from build123d import *

# Parameters (mm, degrees)
CROQUIS1_W              = 190
CROQUIS1_H              = 115.4
SALIENTE_EXTRUIR1_DEPTH = 3
CROQUIS2_R              = 1.6
CORTAR_EXTRUIR1_DEPTH   = 5
CROQUIS4_R              = 1.1
CORTAR_EXTRUIR3_DEPTH   = 5
CROQUIS5_W              = 35.625
CROQUIS5_H              = 40
CORTAR_EXTRUIR4_DEPTH   = 5
REDONDEO1_R             = 3
REDONDEO2_R             = 3
REDONDEO3_R             = 3
REDONDEO4_R             = 3
CROQUIS7_R              = 1.6
CORTAR_EXTRUIR6_DEPTH   = 10
CROQUIS6_R              = 2.1
CORTAR_EXTRUIR7_DEPTH   = 3


with BuildPart() as part:
    # Croquis1 → Saliente-Extruir1 (new body)
    with BuildSketch(Plane(origin=(0, 0, 0), x_dir=(1, 0, 0), z_dir=(0, 1, 0))):
        Rectangle(CROQUIS1_W, CROQUIS1_H)
    extrude(amount=SALIENTE_EXTRUIR1_DEPTH)

    # Croquis2 → Cortar-Extruir1 (cut)
    with BuildSketch(Plane(origin=(0, 3, 0), x_dir=(1, 0, 0), z_dir=(0, 1, 0))):
        with Locations(Location((-36.375, -51.1, 0), (0, 0, 270))):
            Circle(CROQUIS2_R)
        with Locations(Location((-36.375, -10.3, 0), (0, 0, 270))):
            Circle(CROQUIS2_R)
        with Locations(Location((34.375, -10.3, 0), (0, 0, 270))):
            Circle(CROQUIS2_R)
        with Locations(Location((34.375, -51.1, 0), (0, 0, 270))):
            Circle(CROQUIS2_R)
    extrude(amount=-CORTAR_EXTRUIR1_DEPTH, mode=Mode.SUBTRACT)

    # Croquis4 → Cortar-Extruir3 (cut)
    with BuildSketch(Plane(origin=(0, 3, 0), x_dir=(1, 0, 0), z_dir=(0, 1, 0))):
        with Locations(Location((-51.375, -50.7, 0), (0, 0, 270))):
            Circle(CROQUIS4_R)
        with Locations(Location((-51.375, -33.3, 0), (0, 0, 270))):
            Circle(CROQUIS4_R)
        with Locations(Location((51.375, -33.3, 0), (0, 0, 270))):
            Circle(CROQUIS4_R)
        with Locations(Location((51.375, -50.7, 0), (0, 0, 270))):
            Circle(CROQUIS4_R)
    extrude(amount=-CORTAR_EXTRUIR3_DEPTH, mode=Mode.SUBTRACT)

    # Croquis5 → Cortar-Extruir4 (cut)
    with BuildSketch(Plane(origin=(0, 3, 0), x_dir=(1, 0, 0), z_dir=(0, 1, 0))):
        with Locations((-77.1875, -37.7)):
            Rectangle(CROQUIS5_W, CROQUIS5_H)
        Polygon((-95, 57.7), (-95, -17.7), (-59.375, -17.7), (-55, -17.7), (-55, 57.7), align=None)
        with Locations((77.1875, -37.7)):
            Rectangle(CROQUIS5_W, CROQUIS5_H)
        Polygon((55, -17.7), (59.375, -17.7), (95, -17.7), (95, 57.7), (55, 57.7), align=None)
    extrude(amount=-CORTAR_EXTRUIR4_DEPTH, mode=Mode.SUBTRACT)

    # Redondeo1
    redondeo1_edges = [part.edges().sort_by_distance(p)[0] for p in [
        (59.375, 1.5, 17.7),
    ]]
    fillet(redondeo1_edges, radius=REDONDEO1_R)

    # Redondeo2
    redondeo2_edges = [part.edges().sort_by_distance(p)[0] for p in [
        (-59.375, 1.5, 17.7),
    ]]
    fillet(redondeo2_edges, radius=REDONDEO2_R)

    # Redondeo3
    redondeo3_edges = [part.edges().sort_by_distance(p)[0] for p in [
        (-59.375, 1.5, 57.7),
    ]]
    fillet(redondeo3_edges, radius=REDONDEO3_R)

    # Redondeo4
    redondeo4_edges = [part.edges().sort_by_distance(p)[0] for p in [
        (59.375, 1.5, 57.7),
    ]]
    fillet(redondeo4_edges, radius=REDONDEO4_R)

    # Croquis7 → Cortar-Extruir6 (cut)
    with BuildSketch(Plane(origin=(0, 3, 0), x_dir=(1, 0, 0), z_dir=(0, 1, 0))):
        with Locations(Location((27.6, 17, 0), (0, 0, 270))):
            Circle(CROQUIS7_R)
        with Locations(Location((-27.6, 17, 0), (0, 0, 270))):
            Circle(CROQUIS7_R)
        with Locations(Location((-27.6, 37, 0), (0, 0, 270))):
            Circle(CROQUIS7_R)
        with Locations(Location((27.6, 37, 0), (0, 0, 270))):
            Circle(CROQUIS7_R)
    extrude(amount=-CORTAR_EXTRUIR6_DEPTH, mode=Mode.SUBTRACT)

    # Croquis6 → Cortar-Extruir7 (cut)
    with BuildSketch(Plane(origin=(0, 3, 0), x_dir=(1, 0, 0), z_dir=(0, 1, 0))):
        with Locations(Location((-50, 2.7, 0), (0, 0, 270))):
            Circle(CROQUIS6_R)
        with Locations(Location((-50, 12.7, 0), (0, 0, 270))):
            Circle(CROQUIS6_R)
        with Locations(Location((-50, 22.7, 0), (0, 0, 270))):
            Circle(CROQUIS6_R)
        with Locations(Location((-50, 32.7, 0), (0, 0, 270))):
            Circle(CROQUIS6_R)
        with Locations(Location((-50, 42.7, 0), (0, 0, 270))):
            Circle(CROQUIS6_R)
        with Locations(Location((-50, 52.7, 0), (0, 0, 270))):
            Circle(CROQUIS6_R)
        with Locations(Location((50, 2.7, 0), (0, 0, 270))):
            Circle(CROQUIS6_R)
        with Locations(Location((50, 12.7, 0), (0, 0, 270))):
            Circle(CROQUIS6_R)
        with Locations(Location((50, 22.7, 0), (0, 0, 270))):
            Circle(CROQUIS6_R)
        with Locations(Location((50, 32.7, 0), (0, 0, 270))):
            Circle(CROQUIS6_R)
        with Locations(Location((50, 42.7, 0), (0, 0, 270))):
            Circle(CROQUIS6_R)
        with Locations(Location((50, 52.7, 0), (0, 0, 270))):
            Circle(CROQUIS6_R)
    extrude(amount=-CORTAR_EXTRUIR7_DEPTH, mode=Mode.SUBTRACT)


solid = part.part
Work out the finished part from the listing and answer in its coordinate system (mm). Round coordinates to 2 decimals unless told otherwise and drop trailing zeros. Loops run counter-clockwise (first coordinate to the right, second up) from the corner with the lowest first, then second, coordinate; pieces in that order, holes last. Notation, with made-up numbers: (-18, -33.75) - (0, -33.75) arc R19 cw to (0, -0.75) - close; hole circle Ø6 at (-30, 26.5). An arc over 180 degrees is marked (long way). One line per item, written item: value.
Q1. Find section A-A on z = -42.7. Give the vertices of the cut face in (x, y).
Check values:
outline: (-55, 0) - (-52.1, 0) - (-52.1, 3) - (-55, 3) - close; (-47.9, 0) - (47.9, 0) - (47.9, 3) - (-47.9, 3) - close; (52.1, 0) - (55, 0) - (55, 3) - (52.1, 3) - close
Q2. Each of these flat-tipped pins is pushed along its axis until it touches: pin 1 Ø3 at (x, z) = (34.375, 51.1) entering from +Y; pin 2 Ø1 at (y, z) = (2, -43) entering from -X. Where does it stop, or does it pass through?
Check values:
pin 1: through
pin 2: x = -55
Q3. Straight lines are drawn through the part: probe 1 along X at (y, z) = (1.7, -32.7); probe 2 along X at (y, z) = (1.6, 10.3) (3 decimals); probe 3 along Z at (x, y) = (-27, 2.75). For each, find the intervals that lie inside material, in ascending order.
Check values:
probe 1: -55 to -52.1, -47.9 to 47.9, 52.1 to 55
probe 2: -55 to -37.975, -34.775 to 32.775, 35.975 to 55
probe 3: -57.7 to -38.48, -35.52 to -18.48, -15.52 to 57.7
Q4. Find section C-C on y = 0.9. State how many separate pieces and enclosed holes the cut face has, and give its area (3 significant figures).
Check values:
separate pieces: 1
enclosed holes: 24
area: 12,800 mm2
Q5. Find section B-B on x = -27.6. Give the vertices of the cut face in (y, z).
Check values:
outline: (0, -57.7) - (3, -57.7) - (3, -38.6) - (0, -38.6) - close; (0, -35.4) - (3, -35.4) - (3, -18.6) - (0, -18.6) - close; (0, -15.4) - (3, -15.4) - (3, 57.7) - (0, 57.7) - close
Q6. The mould has two halves that part along X. Classify faces 1 (the flat face through (59.375, 2, 38)), 2 (the cylindrical face through (48.722, 1.521, -44.366)), 3 (the flat face through (-59.375, 2, 38)), 4 (the flat face through (-1, 0, -1)): +X half, -X half, draft (parallel to the pull), parting line (faces both ways), or undercut.
Check values:
face 1: +X half
face 2: undercut
face 3: -X half
face 4: draft
